Work out the finished part from the listing and answer in its coordinate system (mm). Coordinates: 2 decimals unless noted, no trailing zeros. Write each loop counter-clockwise with the first axis right and the second up, starting at its lowest first coordinate (ties: lowest second). Pieces come first, ordered by that corner, then holes. Notation, with made-up numbers: (35, -8) - (68, -8) arc R22 cw to (68, 11) - close; hole circle Ø11 at (36.5, 12.5). An arc over 180 degrees is marked (long way). One line per item, written item: value.
```python
from build123d import *

# Parameters (mm, degrees)
AUFSATZ_LINEAR_AUSTRAGEN1_DEPTH = 4
VERRUNDUNG1_R                   = 0.5


with BuildPart() as part:
    # Skizze1 → Aufsatz-Linear austragen1 (new body)
    with BuildSketch(Plane.XY):
        with BuildLine():
            Line((0, 0), (25, 1.53e-15))
            ThreePointArc((25, 1.53e-15), (7.322330470336308, 7.322330470336315), (0, 25))
            Line((0, 25), (0, 0))
        make_face()
    extrude(amount=AUFSATZ_LINEAR_AUSTRAGEN1_DEPTH)

    # Verrundung1
    verrundung1_edges = [part.edges().sort_by_distance(p)[0] for p in [
        (0, 25, 2),
        (25, -1.01e-15, 2),
    ]]
    fillet(verrundung1_edges, radius=VERRUNDUNG1_R - 0.0001)  # a hair under: the kernel refuses the full size


solid = part.part
```
Item 1: Section A-A, the plane x = 8.25 is taken. Determine the outline of the cut face in (y, z), then the cut area to 3 significant figures.
Evaluation:
outline: (0, 0) - (6.44, 0) - (6.44, 4) - (0, 4) - close
area: 25.8 mm2
Item 2: Consider probe 1 along X at (y, z) = (16.5, 3.2); probe 2 along Y at (x, z) = (12.5, 3.65); probe 3 along X at (y, z) = (4, 0.9). Determine where each line is inside the solid, lowest interval first.
Evaluation:
probe 1: x = 0 to 1.49
probe 2: y = 0 to 3.35
probe 3: x = 0 to 11.44
Item 3: Section B-B, the plane y = 17.5 is taken. Determine the outline of the cut face in (x, z), then the cut area to 3 significant figures.
Evaluation:
outline: (0, 0) - (1.15, 0) - (1.15, 4) - (0, 4) - close
area: 4.61 mm2
Item 4: Determine the mould class of faces 1 (the face through (5, 5, 4)), 2 (the face through (5, 5, 0)), 3 (the face through (9, 0, 2)) for opening direction Z: +Z half, -Z half, draft (parallel to the pull), parting line (faces both ways), or undercut.
Evaluation:
face 1: +Z half
face 2: -Z half
face 3: draft
